Work out the finished part from the listing and answer in its coordinate system (mm). Give positions to 0.01 mm unless a question says otherwise; leave off trailing zeros. Order: outer loops, then holes, each group sorted by start corner. A loop starts at its lowest first (then second) coordinate and runs counter-clockwise, first axis right, second up.
```python
from build123d import *

# Parameters (mm, degrees)
SKETCH1_W           = 431.8
SKETCH1_H           = 38.1
BOSS_EXTRUDE1_DEPTH = 6.35
CUT_EXTRUDE1_DEPTH  = 434.524131393
FILLET1_R           = 1.5875


with BuildPart() as part:
    # Sketch1 → Boss-Extrude1 (new body)
    with BuildSketch(Plane.XY):
        with Locations((215.9, 19.05)):
            Rectangle(SKETCH1_W, SKETCH1_H)
    extrude(amount=BOSS_EXTRUDE1_DEPTH)

    # Sketch3 → Cut-Extrude1 (cut, through all)
    with BuildSketch(Plane.XY.offset(6.35)):
        Polygon((75.827293092, 19.05), (9.525, 25.385537758), (9.525, 12.714462242), align=None)
        Polygon((175.507756818, 28.575), (42.903170633, 28.575), (109.205463726, 22.239462242), align=None)
        Polygon((175.507756818, 9.525), (109.205463726, 15.860537758), (42.903170633, 9.525), align=None)
        Polygon((208.885927451, 25.385537758), (142.583634359, 19.05), (208.885927451, 12.714462242), align=None)
        Polygon((289.216365641, 19.05), (222.914072549, 25.385537758), (222.914072549, 12.714462242), align=None)
        Polygon((388.896829367, 28.575), (256.292243182, 28.575), (322.594536274, 22.239462242), align=None)
        Polygon((322.594536274, 15.860537758), (256.292243182, 9.525), (388.896829367, 9.525), align=None)
        Polygon((422.275, 25.385537758), (355.972706908, 19.05), (422.275, 12.714462242), align=None)
    extrude(amount=-CUT_EXTRUDE1_DEPTH, mode=Mode.SUBTRACT)

    # Fillet1
    fillet1_edges = [part.edges().sort_by_distance(p)[0] for p in [
        (289.216365641, 19.05, 3.175),
        (222.914072549, 12.714462242, 3.175),
        (222.914072549, 25.385537758, 3.175),
        (142.583634359, 19.05, 3.175),
        (208.885927451, 25.385537758, 3.175),
        (208.885927451, 12.714462242, 3.175),
        (42.903170633, 9.525, 3.175),
        (109.205463726, 15.860537758, 3.175),
        (175.507756818, 9.525, 3.175),
        (109.205463726, 22.239462242, 3.175),
        (42.903170633, 28.575, 3.175),
        (175.507756818, 28.575, 3.175),
        (422.275, 25.385537758, 3.175),
        (422.275, 12.714462242, 3.175),
        (355.972706908, 19.05, 3.175),
        (322.594536274, 15.860537758, 3.175),
        (388.896829367, 9.525, 3.175),
        (256.292243182, 9.525, 3.175),
        (388.896829367, 28.575, 3.175),
        (322.594536274, 22.239462242, 3.175),
        (256.292243182, 28.575, 3.175),
        (9.525, 12.714462242, 3.175),
        (9.525, 25.385537758, 3.175),
        (75.827293092, 19.05, 3.175),
    ]]
    fillet(fillet1_edges, radius=FILLET1_R)


solid = part.part
```
1. The part is cut by section B-B (z = 4.5). State how many separate pieces and enclosed holes the cut face has, then the cut area to 3 significant figures.
Findings below:
separate pieces: 1
enclosed holes: 8
area: 13,600 mm2
2. The part is cut by section A-A (x = 132.5). Write down the section's boundary in (y, z) (3 decimals), then the cut area to 3 significant figures.
Findings below:
outline: (0, 0) - (9.525, 0) - (9.525, 6.35) - (0, 6.35) - close; (13.635, 0) - (24.465, 0) - (24.465, 6.35) - (13.635, 6.35) - close; (28.575, 0) - (38.1, 0) - (38.1, 6.35) - (28.575, 6.35) - close
area: 190 mm2
3. Straight lines are drawn through the part: probe 1 along X at (y, z) = (19.5, 3.75) (3 decimals); probe 2 along Y at (x, z) = (289.5, 1); probe 3 along Y at (x, z) = (390, 0.75). For each, find the intervals that lie inside material, in ascending order.
Findings below:
probe 1: x = 0 to 9.525, 60.661 to 157.75, 208.886 to 222.914, 274.05 to 371.139, 422.275 to 431.8
probe 2: y = 0 to 9.53, 12.7 to 25.4, 28.57 to 38.1
probe 3: y = 0 to 15.8, 22.3 to 38.1
4. The part is cut by section C-C (x = 190). Write down the section's boundary in (y, z), then the cut area to 3 significant figures.
Findings below:
outline: (0, 0) - (14.52, 0) - (14.52, 6.35) - (0, 6.35) - close; (23.58, 0) - (38.1, 0) - (38.1, 6.35) - (23.58, 6.35) - close
area: 184 mm2
